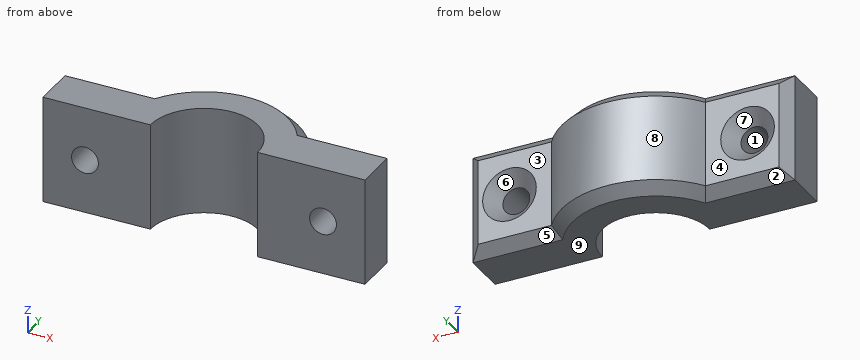
Autodesk Fusion 360 part; units mm, degrees
sketch "Sketch1" plane through (0, 0, 0) normal (0, 0, 1) x (1, 0, 0)
  line L0 (-10, 0) -> (-30, 0)
  line L1 (10, 0) -> (30, 0)
  line L2 (-30, 0) -> (-30, 10)
  line L3 (30, 0) -> (30, 10)
  arc A0 (14.3614, 10) -> (-14.3614, 10) centre (0, 0) ccw
  line L4 (-30, 10) -> (-14.3614, 10)
  line L5 (14.3614, 10) -> (30, 10)
  arc A1 (10, 0) -> (-10, 0) centre (0, 0) ccw
  dimension "d1" = 20
  dimension "d2" = 35
extrude "Extrude1" add sketch "Sketch1" along normal blind 20
sketch "Sketch2" plane through (0, 10, 0) normal (0, 1, 0) x (-1, 0, 0)
  line L0 (-30, 0) -> (-14.3614, 0)
  line L1 (-14.3614, 0) -> (-14.3614, 20)
  line L2 (-14.3614, 20) -> (-30, 20)
  line L3 (-30, 20) -> (-30, 0)
  line L4 (-30, 20) -> (-14.3614, 0)
  line L5 (-14.3614, 20) -> (-30, 0)
hole "Hole1" at (22.1807, 10, 10) direction (0, -1, 0) diameter 5 depth 10 tip angle 118 countersink diameter 10 countersink angle 90
sketch "Sketch3" plane through (0, 10, 0) normal (0, 1, 0) x (-1, 0, 0)
  line L0 (14.3614, 0) -> (30, 0)
  line L1 (30, 0) -> (30, 20)
  line L2 (30, 20) -> (14.3614, 20)
  line L3 (14.3614, 20) -> (14.3614, 0)
  line L4 (14.3614, 20) -> (30, 0)
  line L5 (14.3614, 0) -> (30, 20)
hole "Hole2" at (-22.1807, 10, 10) direction (0, -1, 0) diameter 5 depth 10 tip angle 118 countersink diameter 10 countersink angle 90
chamfer "Chamfer1" distance 2 angle 45 8 edges at (-30, 10, 10) (30, 10, 10) (22.1807, 10, 0) (-22.1807, 10, 0) (-22.1807, 10, 20) (22.1807, 10, 20) (0, 17.5, 20) (0, 17.5, 0)
Can you work these out from the model? Positions are in its coordinate system, mm. Face numbers are marked on the shaded views. A direction names the side the tool comes from. Give positions to 0.01 mm unless a question says otherwise; leave off trailing zeros. Loops run counter-clockwise (first coordinate to the right, second up) from the corner with the lowest first, then second, coordinate; pieces in that order, holes last. Notation, with made-up numbers: (86.25, 76) - (131.25, 76) arc R18 cw to (131.25, 103) - close; hole circle Ø8 at (76.25, 0). An arc over 180 degrees is marked (long way). One line per item, written item: value.
(1) If we mould it in two halves opening along Z, with no side actions, what happens to the marked faces 6, 7, 8 and 9? For each: released by +Z, released by -Z, zero draft, split by the parting line, or undercut.
Verdict:
face 6: undercut
face 7: undercut
face 8: zero draft
face 9: released by -Z
(2) On a 3-axis mill with a long thin cutter (end or side, diameter ignored), from which of +Z, -Z, +X, -X, +Y, -Y can I reach the whole of each face in a straight line? I mean the marked faces 1, 2, 3, 4 and 5. Say none if no direction works.
Verdict:
face 1: +Y, -Y
face 2: -Z, -X, +Y
face 3: +Z, -Z, +X, +Y
face 4: +Z, -Z, -X, +Y
face 5: -Z, +X, +Y
(3) If we section it at C-C, the plane x = 0: List the corners of the cut face in (y, z) for me, plus the area to 3 significant figures.
Verdict:
outline: (10, 0) - (15.5, 0) - (17.5, 2) - (17.5, 18) - (15.5, 20) - (10, 20) - close
area: 146 mm^2
(4) If we section it at D-D, the plane y = 3.5: List the corners of the cut face in (x, z) for me, plus the area to 3 significant figures.
Verdict:
outline: (-30, 0) - (-9.37, 0) - (-9.37, 20) - (-30, 20) - close; (9.37, 0) - (30, 0) - (30, 20) - (9.37, 20) - close; hole circle Ø5 at (-22.18, 10); hole circle Ø5 at (22.18, 10)
area: 786 mm^2
(5) I need wall thicknesses on line 1 along X through (y, z) = (1.75, 10); line 2 along X through (y, z) = (6.25, 12); line 3 along Y through (x, z) = (15.5, 7). Which ranges of each line are inside material? Lowest first, please.
Verdict:
line 1: -30 to -24.68, -19.68 to -9.85, 9.85 to 19.68, 24.68 to 30
line 2: -30 to -23.68, -20.68 to -7.81, 7.81 to 20.68, 23.68 to 30
line 3: 0 to 10
(6) If we section it at A-A, the plane z = 10: List the corners of the cut face in (x, y) for me, plus the area to 3 significant figures.
Verdict:
outline: (-30, 0) - (-24.68, 0) - (-24.68, 7.5) - (-27.18, 10) - (-28, 10) - (-30, 8) - close; (-19.68, 0) - (-10, 0) arc R10 cw to (10, 0) - (19.68, 0) - (19.68, 7.5) - (17.18, 10) - (14.36, 10) arc R17.5 ccw to (-14.36, 10) - (-17.18, 10) - (-19.68, 7.5) - close; (24.68, 0) - (30, 0) - (30, 8) - (28, 10) - (27.18, 10) - (24.68, 7.5) - close
area: 478 mm^2
(7) I'm going to push flat-ended pins straight in: pin 1 (4 mm diameter, centred on x = 22.5, z = 11, fed in from +Y); pin 2 (5 mm diameter, centred on x = 4.5, z = 3.5, fed in from +Y); pin 3 (4 mm diameter, centred on x = -8, z = 13.5, fed in from +Y). Where does each tip first touch, or does it pass through?
Verdict:
pin 1: y = 8.05
pin 2: y = 17.39
pin 3: y = 16.44
(8) If we section it at B-B, the plane y = 6.75: List the corners of the cut face in (x, z) for me.
Verdict:
outline: (-30, 0) - (-7.38, 0) - (-7.38, 20) - (-30, 20) - close; (7.38, 0) - (30, 0) - (30, 20) - (7.38, 20) - close; hole circle Ø5 at (-22.18, 10); hole circle Ø5 at (22.18, 10)
